from build123d import *

# Parameters (mm, degrees)
SKETCH1_W           = 36
SKETCH1_H           = 9
SKETCH1_R           = 1.6
SKETCH1_R_2         = 2.5
BOSS_EXTRUDE1_DEPTH = 2.5
SKETCH2_W           = 8.796746506
SKETCH2_H           = 9
SKETCH2_R           = 2.5
BOSS_EXTRUDE2_DEPTH = 5


with BuildPart() as part:
    # Sketch1 → Boss-Extrude1 (new body)
    with BuildSketch(Plane(origin=(0, 0, 0), x_dir=(1, 0, 0), z_dir=(0, 1, 0))):
        with Locations((-8.854143772, 0)):
            Rectangle(SKETCH1_W, SKETCH1_H)
        with Locations((-13.354143772, 0)):
            Circle(SKETCH1_R, mode=Mode.SUBTRACT)
        with Locations((-4.354143772, 0)):
            Circle(SKETCH1_R, mode=Mode.SUBTRACT)
        with Locations((4.645856228, 0)):
            Circle(SKETCH1_R_2, mode=Mode.SUBTRACT)
        with Locations((-22.354143772, 0)):
            Circle(SKETCH1_R_2, mode=Mode.SUBTRACT)
    extrude(amount=BOSS_EXTRUDE1_DEPTH)

    # Sketch2 → Boss-Extrude2 (add)
    with BuildSketch(Plane(origin=(0, 2.5, 0), x_dir=(1, 0, 0), z_dir=(0, 1, 0))):
        with Locations((-22.455770519, 0)):
            Rectangle(SKETCH2_W, SKETCH2_H)
        with Locations((-22.354143772, 0)):
            Circle(SKETCH2_R, mode=Mode.SUBTRACT)
        with Locations((4.747482975, 0)):
            Rectangle(SKETCH2_W, SKETCH2_H)
        with Locations((4.645856228, 0)):
            Circle(SKETCH2_R, mode=Mode.SUBTRACT)
    extrude(amount=BOSS_EXTRUDE2_DEPTH)


solid = part.part
The listing builds one solid part. Answer for the finished solid, in the listing's coordinates (mm). A direction names the side the tool comes from. Coordinates: 2 decimals unless noted, no trailing zeros. Loops run counter-clockwise (first coordinate to the right, second up) from the corner with the lowest first, then second, coordinate; pieces in that order, holes last.
1) Find section C-C on z = 4. Write down the section's boundary in (x, y).
2) Find the intervals of material crossed by L1, parallel to X at y = 1.4, z = 0; L2, parallel to X at y = 5, z = 0; L3, parallel to X at y = 7, z = -2, in increasing order.
3) A flat-ended cylindrical pin translates along its axis: pin 1 Ø4.5 at (x, z) = (-4.5, 1.5) entering from +Y. Find the tip coordinate at first contact, or state that the pin passes through.
4) Find section A-A on y = 4.25. Write down the section's boundary in (x, z).
5) Determine the mould class of faces 1 (the face through (-9, 2.5, 0)), 2 (the face through (-14.953, 1.232, -0.07)), 3 (the face through (-9, 2, -4.5)) for opening direction Z: pulls with the +Z half, pulls with the -Z half, needs draft (parallel to the pull), parting line crosses it, or undercut.
6) A tool of negligible diameter and unlimited length cuts with its end or side. For faces 4 (the face through (-20.045, 3.698, 0.958)), 5 (the face through (0.349, 5, 0)), from which of +Z, -Z, +X, -X, +Y, -Y can it reach the whole face along a straight path? Write none if from no direction.
7) Find section B-B on z = -0.5. Write down the section's boundary in (x, y), then the cut area to 3 significant figures.
Values:
1. outline: (-26.85, 0) - (9.15, 0) - (9.15, 7.5) - (0.35, 7.5) - (0.35, 2.5) - (-18.06, 2.5) - (-18.06, 7.5) - (-26.85, 7.5) - close
2. L1: x = -26.85 to -24.85, -19.85 to -14.95, -11.75 to -5.95, -2.75 to 2.15, 7.15 to 9.15
2. L2: x = -26.85 to -24.85, -19.85 to -18.06, 0.35 to 2.15, 7.15 to 9.15
2. L3: x = -26.85 to -23.85, -20.85 to -18.06, 0.35 to 3.15, 6.15 to 9.15
3. pin 1: stops at y = 2.5
4. outline: (-26.85, -4.5) - (-18.06, -4.5) - (-18.06, 4.5) - (-26.85, 4.5) - close; (0.35, -4.5) - (9.15, -4.5) - (9.15, 4.5) - (0.35, 4.5) - close; hole circle Ø5 at (-22.35, 0); hole circle Ø5 at (4.65, 0)
5. face 1: needs draft
5. face 2: undercut
5. face 3: pulls with the -Z half
6. face 4: +Y, -Y
6. face 5: +Z, -Z, +Y
7. outline: (-26.85, 0) - (-24.8, 0) - (-24.8, 7.5) - (-26.85, 7.5) - close; (-19.9, 0) - (-14.87, 0) - (-14.87, 2.5) - (-18.06, 2.5) - (-18.06, 7.5) - (-19.9, 7.5) - close; (-11.83, 0) - (-5.87, 0) - (-5.87, 2.5) - (-11.83, 2.5) - close; (-2.83, 0) - (2.2, 0) - (2.2, 7.5) - (0.35, 7.5) - (0.35, 2.5) - (-2.83, 2.5) - close; (7.1, 0) - (9.15, 0) - (9.15, 7.5) - (7.1, 7.5) - close
7. area: 89.3 mm2
